Work out the finished part from the listing and answer in its coordinate system (mm). Face numbers are marked on the shaded views. A direction names the side the tool comes from. Round coordinates to 2 decimals unless told otherwise and drop trailing zeros. Write each loop counter-clockwise with the first axis right and the second up, starting at its lowest first coordinate (ties: lowest second). Pieces come first, ordered by that corner, then holes. Notation, with made-up numbers: (1.25, 86.25) - (42.25, 86.25) arc R34 ccw to (42.25, 122.25) - close; hole circle Ø9 at (-26.75, 31). An arc over 180 degrees is marked (long way). Answer as a JSON object with one key per item and string values.
```python
from build123d import *

# Parameters (mm, degrees)
CUT_EXTRUDE1_START       = -22.385915399
CUT_EXTRUDE1_OUTLINE_R   = 1.85
CUT_EXTRUDE1_DEPTH       = 4
CUT_EXTRUDE1_START_2     = -18.385915399
CUT_EXTRUDE1_2_OUTLINE_R = 1.85
CUT_EXTRUDE1_2_DEPTH     = 40.98
CUT_EXTRUDE1_START_3     = -12.299495873
CUT_EXTRUDE1_3_DEPTH     = 12.7
SKETCH2_W                = 30.48
SKETCH2_H                = 44.98
BOSS_EXTRUDE1_DEPTH      = 6.35
CUT_EXTRUDE2_REACH       = 69.384
SKETCH3_R                = 1.85
BOSS_EXTRUDE3_REACH      = 66.446
SKETCH4_W                = 67.174
SKETCH4_H                = 12.7
SKETCH5_W                = 6.35
SKETCH5_H                = 17.78
BOSS_EXTRUDE4_DEPTH      = 0.1
FILLET1_R                = 3.175


with BuildPart() as part:
    # Cut-Extrude1: read off the stored shape, not the designer's step
    # Cut-Extrude1 outline → Cut-Extrude1 (new body)
    with BuildSketch(Plane(origin=(0, 0, 0), x_dir=(1, 0, 0), z_dir=(0, 1, 0)).offset(CUT_EXTRUDE1_START)):
        with BuildLine():
            ThreePointArc((41.290674946, 5.949495873), (41.56736633, 6.922737878), (42.314674946, 7.604858069))
            Line((42.314674946, 7.604858069), (42.314674946, 12.299495873))
            Line((42.314674946, 12.299495873), (-24.859325054, 12.299495873))
            Line((-24.859325054, 12.299495873), (-24.859325054, -0.400504127))
            Line((-24.859325054, -0.400504127), (42.314674946, -0.400504127))
            Line((42.314674946, -0.400504127), (42.314674946, 4.294133677))
            ThreePointArc((42.314674946, 4.294133677), (41.56736633, 4.976253868), (41.290674946, 5.949495873))
        make_face()
        with Locations((-20.859325054, 5.949495873)):
            Circle(CUT_EXTRUDE1_OUTLINE_R, mode=Mode.SUBTRACT)
    extrude(amount=CUT_EXTRUDE1_DEPTH)

    # Cut-Extrude1 2 outline → Cut-Extrude1 2 (add)
    with BuildSketch(Plane(origin=(0, 0, 0), x_dir=(1, 0, 0), z_dir=(0, 1, 0)).offset(CUT_EXTRUDE1_START_2)):
        with BuildLine():
            ThreePointArc((41.290674946, 5.949495873), (41.56736633, 6.922737878), (42.314674946, 7.604858069))
            Line((42.314674946, 7.604858069), (42.314674946, 12.299495873))
            Line((42.314674946, 12.299495873), (-24.859325054, 12.299495873))
            Line((-24.859325054, 12.299495873), (-24.859325054, -0.400504127))
            Line((-24.859325054, -0.400504127), (42.314674946, -0.400504127))
            Line((42.314674946, -0.400504127), (42.314674946, 4.294133677))
            ThreePointArc((42.314674946, 4.294133677), (41.56736633, 4.976253868), (41.290674946, 5.949495873))
        make_face()
        with Locations((-20.859325054, 5.949495873)):
            Circle(CUT_EXTRUDE1_2_OUTLINE_R, mode=Mode.SUBTRACT)
    extrude(amount=CUT_EXTRUDE1_2_DEPTH)

    # Cut-Extrude1 3 outline → Cut-Extrude1 3 (cut)
    with BuildSketch(Plane.XY.offset(CUT_EXTRUDE1_START_3)):
        with BuildLine():
            Line((-7.298413969, 1.614084601), (-24.859325054, 1.614084601))
            Line((-24.859325054, 1.614084601), (-24.859325054, -1.385915399))
            Line((-24.859325054, -1.385915399), (-7.298413969, -1.385915399))
            ThreePointArc((-7.298413969, -1.385915399), (11.891293051, -18.370681356), (29.640674946, 0.114084601))
            ThreePointArc((29.640674946, 0.114084601), (11.891293051, 18.598850557), (-7.298413969, 1.614084601))
        make_face()
        with BuildLine():
            ThreePointArc((-8.270513308, 11.452345957), (-0.050086584, 19.610680621), (11.140674816, 22.594084601))
            Line((11.140674816, 22.594084601), (-24.859325054, 22.594084601))
            Line((-24.859325054, 22.594084601), (-24.859325054, 6.805102167))
            ThreePointArc((-24.859325054, 6.805102167), (-24.419985226, 7.865762339), (-23.359325054, 8.305102167))
            Line((-23.359325054, 8.305102167), (-13.753655898, 8.305102167))
            ThreePointArc((-13.753655898, 8.305102167), (-10.592564467, 9.147834154), (-8.270513308, 11.452345957))
        make_face()
        with BuildLine():
            Line((39.26266634, 0.114084601), (42.314674946, 0.114084601))
            Line((42.314674946, 0.114084601), (42.314674946, 22.594084601))
            Line((42.314674946, 22.594084601), (11.140674816, 22.594084601))
            ThreePointArc((11.140674816, 22.594084601), (25.177120317, 17.67337278), (33.068609963, 5.065454701))
            ThreePointArc((33.068609963, 5.065454701), (35.297745147, 1.504054366), (39.26266634, 0.114084601))
        make_face()
    extrude(amount=CUT_EXTRUDE1_3_DEPTH, mode=Mode.SUBTRACT)

    # Sketch2 → Boss-Extrude1 (add)
    with BuildSketch(Plane(origin=(42.314674946, 0, 0), x_dir=(0, 0, -1), z_dir=(1, 0, 0))):
        with Locations((-2.940504127, 0.104084601)):
            Rectangle(SKETCH2_W, SKETCH2_H)
    extrude(amount=-BOSS_EXTRUDE1_DEPTH)

    # Sketch3 → Cut-Extrude2 (cut, up to next)
    with BuildSketch(Plane.ZY.offset(-35.964674946), mode=Mode.PRIVATE) as cut_extrude2_sk1:
        with Locations(Location((9.177002591, 16.869259883, 0), (0, 0, 270))):
            Circle(SKETCH3_R)
    cut_extrude2_tool1 = extrude(cut_extrude2_sk1.sketch, amount=-CUT_EXTRUDE2_REACH, mode=Mode.PRIVATE) & part.part
    # Sketch3 → Cut-Extrude2 (cut, up to next)
    with BuildSketch(Plane.ZY.offset(-35.964674946), mode=Mode.PRIVATE) as cut_extrude2_sk2:
        with Locations(Location((9.177002591, 5.863674358, 0), (0, 0, 270))):
            Circle(SKETCH3_R)
    cut_extrude2_tool2 = extrude(cut_extrude2_sk2.sketch, amount=-CUT_EXTRUDE2_REACH, mode=Mode.PRIVATE) & part.part
    # Sketch3 → Cut-Extrude2 (cut, up to next)
    with BuildSketch(Plane.ZY.offset(-35.964674946), mode=Mode.PRIVATE) as cut_extrude2_sk3:
        with Locations(Location((9.177002591, -13.873009015, 0), (0, 0, 270))):
            Circle(SKETCH3_R)
    cut_extrude2_tool3 = extrude(cut_extrude2_sk3.sketch, amount=-CUT_EXTRUDE2_REACH, mode=Mode.PRIVATE) & part.part
    add(cut_extrude2_tool1.solids().sort_by_distance((35.964675, 16.86926, 9.177003))[0], mode=Mode.SUBTRACT)
    add(cut_extrude2_tool2.solids().sort_by_distance((35.964675, 5.863674, 9.177003))[0], mode=Mode.SUBTRACT)
    add(cut_extrude2_tool3.solids().sort_by_distance((35.964675, -13.873009, 9.177003))[0], mode=Mode.SUBTRACT)

    # Sketch4 → Boss-Extrude3 (add, up to next)
    with BuildSketch(Plane(origin=(0, 22.694084601, 0), x_dir=(1, 0, 0), z_dir=(0, 1, 0)), mode=Mode.PRIVATE) as boss_extrude3_sk1:
        with Locations((8.727674946, 5.949495873)):
            Rectangle(SKETCH4_W, SKETCH4_H)
        with BuildLine():
            ThreePointArc((-19.009325054, 5.949495873), (-20.859325054, 7.799495873), (-22.709325054, 5.949495873))
            ThreePointArc((-22.709325054, 5.949495873), (-20.859325054, 4.099495873), (-19.009325054, 5.949495873))
        make_face(mode=Mode.SUBTRACT)
    boss_extrude3_tool1 = extrude(boss_extrude3_sk1.sketch, amount=-BOSS_EXTRUDE3_REACH, mode=Mode.PRIVATE) - part.part
    add(boss_extrude3_tool1.solids().sort_by_distance((9.105332, 22.694085, -5.949496))[0])

    # Sketch5 → Boss-Extrude4 (add)
    with BuildSketch(Plane(origin=(0, 22.594084601, 0), x_dir=(1, 0, 0), z_dir=(0, 1, 0))):
        with Locations((39.139674946, -9.290504127)):
            Rectangle(SKETCH5_W, SKETCH5_H)
    extrude(amount=BOSS_EXTRUDE4_DEPTH)

    # Fillet1
    fillet1_edges = [part.edges().sort_by_distance(p)[0] for p in [
        (35.964674946, -10.674112441, 0.400504127),
    ]]
    fillet(fillet1_edges, radius=FILLET1_R)


solid = part.part
```
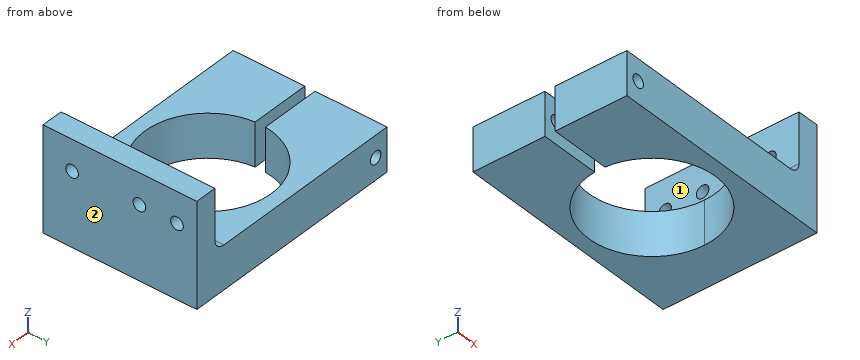
Item 1: A cutting plane is placed at A-A (x = -13). Write down the section's boundary in (y, z).
Results found:
{"outline": "(-22.39, -12.3) - (-1.39, -12.3) - (-1.39, 0.4) - (-22.39, 0.4) - close; (1.61, -12.3) - (22.69, -12.3) - (22.69, 0.4) - (1.61, 0.4) - close"}
Item 2: A cutting plane is placed at C-C (z = -1.5). Write down the section's boundary in (x, y), and give its area (3 significant figures).
Results found:
{"outline": "(-24.86, -22.39) - (42.31, -22.39) - (42.31, 22.69) - (-24.86, 22.69) - (-24.86, 1.61) - (-7.3, 1.61) arc R18.5 cw (long way) to (-7.3, -1.39) - (-24.86, -1.39) - close", "area": "1,900 mm²"}
Item 3: Each of these flat-tipped pins is pushed along its axis until it touches: P1, Ø2, axis at x = 28, y = -12, coming from the +Z side; P2, Ø7.5, axis at y = -3, z = 10.5, coming from the -X side. Where does it stop, or does it pass through?
Results found:
{"P1": "z = 0.4", "P2": "x = 35.96"}
Item 4: A cutting plane is placed at B-B (y = -17). Give the number of separate pieces and of enclosed holes in the cut face, and give its area (3 significant figures).
Results found:
{"separate pieces": "2", "enclosed holes": "1", "area": "779 mm²"}
Item 5: For the marked faces 1 and 2, determine the directions among +Z, -Z, +X, -X, +Y, -Y from which every point of the face is accessible in a straight line to the end or side of a thin tool.
Results found:
{"face 1": "+Z, -X, +Y, -Y", "face 2": "+Z, -Z, +X, +Y, -Y"}
Item 6: Consider line 1 along X through (y, z) = (-8, -7); line 2 along Y through (x, z) = (36.5, 9.5); line 3 along X through (y, z) = (-13, -7.5). Determine where each line is inside the solid, lowest interval first.
Results found:
{"line 1": "-24.86 to -22.38, -19.34 to -5.48, 27.77 to 42.31", "line 2": "-22.39 to -15.69, -12.05 to 4.04, 7.69 to 15.05, 18.69 to 22.69", "line 3": "-24.86 to -21.87, -19.85 to -1.91, 24.19 to 42.31"}
